from build123d import *

# Parameters (mm, degrees)
IZIM1_W                     = 500
IZIM1_H                     = 300
Y_KSEKLIK_EKSTR_ZYON1_DEPTH = 3


with BuildPart() as part:
    # Çizim1 → Yükseklik-Ekstrüzyon1 (new body)
    with BuildSketch(Plane.XY):
        with Locations((250, -150)):
            Rectangle(IZIM1_W, IZIM1_H)
        with BuildLine():
            Line((50, -40), (50, -120))
            ThreePointArc((50, -120), (45, -125), (40, -120))
            Line((40, -120), (40, -40))
            ThreePointArc((40, -40), (45, -35), (50, -40))
        make_face(mode=Mode.SUBTRACT)
        with BuildLine():
            Line((87.272727273, -40), (87.272727273, -120))
            ThreePointArc((87.272727273, -120), (82.272727273, -125), (77.272727273, -120))
            Line((77.272727273, -120), (77.272727273, -40))
            ThreePointArc((77.272727273, -40), (82.272727273, -35), (87.272727273, -40))
        make_face(mode=Mode.SUBTRACT)
        with BuildLine():
            Line((124.545454545, -40), (124.545454545, -120))
            ThreePointArc((124.545454545, -120), (119.545454545, -125), (114.545454545, -120))
            Line((114.545454545, -120), (114.545454545, -40))
            ThreePointArc((114.545454545, -40), (119.545454545, -35), (124.545454545, -40))
        make_face(mode=Mode.SUBTRACT)
        with BuildLine():
            Line((161.818181818, -40), (161.818181818, -120))
            ThreePointArc((161.818181818, -120), (156.818181818, -125), (151.818181818, -120))
            Line((151.818181818, -120), (151.818181818, -40))
            ThreePointArc((151.818181818, -40), (156.818181818, -35), (161.818181818, -40))
        make_face(mode=Mode.SUBTRACT)
        with BuildLine():
            Line((199.090909091, -40), (199.090909091, -120))
            ThreePointArc((199.090909091, -120), (194.090909091, -125), (189.090909091, -120))
            Line((189.090909091, -120), (189.090909091, -40))
            ThreePointArc((189.090909091, -40), (194.090909091, -35), (199.090909091, -40))
        make_face(mode=Mode.SUBTRACT)
        with BuildLine():
            Line((236.363636364, -40), (236.363636364, -120))
            ThreePointArc((236.363636364, -120), (231.363636364, -125), (226.363636364, -120))
            Line((226.363636364, -120), (226.363636364, -40))
            ThreePointArc((226.363636364, -40), (231.363636364, -35), (236.363636364, -40))
        make_face(mode=Mode.SUBTRACT)
        with BuildLine():
            Line((273.636363636, -40), (273.636363636, -120))
            ThreePointArc((273.636363636, -120), (268.636363636, -125), (263.636363636, -120))
            Line((263.636363636, -120), (263.636363636, -40))
            ThreePointArc((263.636363636, -40), (268.636363636, -35), (273.636363636, -40))
        make_face(mode=Mode.SUBTRACT)
        with BuildLine():
            Line((310.909090909, -40), (310.909090909, -120))
            ThreePointArc((310.909090909, -120), (305.909090909, -125), (300.909090909, -120))
            Line((300.909090909, -120), (300.909090909, -40))
            ThreePointArc((300.909090909, -40), (305.909090909, -35), (310.909090909, -40))
        make_face(mode=Mode.SUBTRACT)
        with BuildLine():
            Line((348.181818182, -40), (348.181818182, -120))
            ThreePointArc((348.181818182, -120), (343.181818182, -125), (338.181818182, -120))
            Line((338.181818182, -120), (338.181818182, -40))
            ThreePointArc((338.181818182, -40), (343.181818182, -35), (348.181818182, -40))
        make_face(mode=Mode.SUBTRACT)
        with BuildLine():
            Line((385.454545455, -40), (385.454545455, -120))
            ThreePointArc((385.454545455, -120), (380.454545455, -125), (375.454545455, -120))
            Line((375.454545455, -120), (375.454545455, -40))
            ThreePointArc((375.454545455, -40), (380.454545455, -35), (385.454545455, -40))
        make_face(mode=Mode.SUBTRACT)
        with BuildLine():
            Line((422.727272727, -40), (422.727272727, -120))
            ThreePointArc((422.727272727, -120), (417.727272727, -125), (412.727272727, -120))
            Line((412.727272727, -120), (412.727272727, -40))
            ThreePointArc((412.727272727, -40), (417.727272727, -35), (422.727272727, -40))
        make_face(mode=Mode.SUBTRACT)
        with BuildLine():
            Line((460, -40), (460, -120))
            ThreePointArc((460, -120), (455, -125), (450, -120))
            Line((450, -120), (450, -40))
            ThreePointArc((450, -40), (455, -35), (460, -40))
        make_face(mode=Mode.SUBTRACT)
        with BuildLine():
            Line((87.272727273, -180), (87.272727273, -260))
            ThreePointArc((87.272727273, -260), (82.272727273, -265), (77.272727273, -260))
            Line((77.272727273, -260), (77.272727273, -180))
            ThreePointArc((77.272727273, -180), (82.272727273, -175), (87.272727273, -180))
        make_face(mode=Mode.SUBTRACT)
        with BuildLine():
            Line((124.545454545, -180), (124.545454545, -260))
            ThreePointArc((124.545454545, -260), (119.545454545, -265), (114.545454545, -260))
            Line((114.545454545, -260), (114.545454545, -180))
            ThreePointArc((114.545454545, -180), (119.545454545, -175), (124.545454545, -180))
        make_face(mode=Mode.SUBTRACT)
        with BuildLine():
            Line((161.818181818, -180), (161.818181818, -260))
            ThreePointArc((161.818181818, -260), (156.818181818, -265), (151.818181818, -260))
            Line((151.818181818, -260), (151.818181818, -180))
            ThreePointArc((151.818181818, -180), (156.818181818, -175), (161.818181818, -180))
        make_face(mode=Mode.SUBTRACT)
        with BuildLine():
            Line((199.090909091, -180), (199.090909091, -260))
            ThreePointArc((199.090909091, -260), (194.090909091, -265), (189.090909091, -260))
            Line((189.090909091, -260), (189.090909091, -180))
            ThreePointArc((189.090909091, -180), (194.090909091, -175), (199.090909091, -180))
        make_face(mode=Mode.SUBTRACT)
        with BuildLine():
            Line((236.363636364, -180), (236.363636364, -260))
            ThreePointArc((236.363636364, -260), (231.363636364, -265), (226.363636364, -260))
            Line((226.363636364, -260), (226.363636364, -180))
            ThreePointArc((226.363636364, -180), (231.363636364, -175), (236.363636364, -180))
        make_face(mode=Mode.SUBTRACT)
        with BuildLine():
            Line((273.636363636, -180), (273.636363636, -260))
            ThreePointArc((273.636363636, -260), (268.636363636, -265), (263.636363636, -260))
            Line((263.636363636, -260), (263.636363636, -180))
            ThreePointArc((263.636363636, -180), (268.636363636, -175), (273.636363636, -180))
        make_face(mode=Mode.SUBTRACT)
        with BuildLine():
            Line((310.909090909, -180), (310.909090909, -260))
            ThreePointArc((310.909090909, -260), (305.909090909, -265), (300.909090909, -260))
            Line((300.909090909, -260), (300.909090909, -180))
            ThreePointArc((300.909090909, -180), (305.909090909, -175), (310.909090909, -180))
        make_face(mode=Mode.SUBTRACT)
        with BuildLine():
            Line((348.181818182, -180), (348.181818182, -260))
            ThreePointArc((348.181818182, -260), (343.181818182, -265), (338.181818182, -260))
            Line((338.181818182, -260), (338.181818182, -180))
            ThreePointArc((338.181818182, -180), (343.181818182, -175), (348.181818182, -180))
        make_face(mode=Mode.SUBTRACT)
        with BuildLine():
            Line((385.454545455, -180), (385.454545455, -260))
            ThreePointArc((385.454545455, -260), (380.454545455, -265), (375.454545455, -260))
            Line((375.454545455, -260), (375.454545455, -180))
            ThreePointArc((375.454545455, -180), (380.454545455, -175), (385.454545455, -180))
        make_face(mode=Mode.SUBTRACT)
        with BuildLine():
            Line((422.727272727, -180), (422.727272727, -260))
            ThreePointArc((422.727272727, -260), (417.727272727, -265), (412.727272727, -260))
            Line((412.727272727, -260), (412.727272727, -180))
            ThreePointArc((412.727272727, -180), (417.727272727, -175), (422.727272727, -180))
        make_face(mode=Mode.SUBTRACT)
        with BuildLine():
            Line((460, -180), (460, -260))
            ThreePointArc((460, -260), (455, -265), (450, -260))
            Line((450, -260), (450, -180))
            ThreePointArc((450, -180), (455, -175), (460, -180))
        make_face(mode=Mode.SUBTRACT)
        with BuildLine():
            Line((50, -180), (50, -260))
            ThreePointArc((50, -260), (45, -265), (40, -260))
            Line((40, -260), (40, -180))
            ThreePointArc((40, -180), (45, -175), (50, -180))
        make_face(mode=Mode.SUBTRACT)
    extrude(amount=Y_KSEKLIK_EKSTR_ZYON1_DEPTH)


solid = part.part
Can you work these out from the model? Positions are in its coordinate system, mm. Give positions to 0.01 mm unless a question says otherwise; leave off trailing zeros. Write each loop counter-clockwise with the first axis right and the second up, starting at its lowest first coordinate (ties: lowest second). Pieces come first, ordered by that corner, then holes. Notation, with made-up numbers: M 66.25,15 L 115.25,15 A27 ccw 115.25,43 Z; hole C -34,76.25 d8. An arc over 180 degrees is marked long. Answer in a Markdown table with one row per item. Add a question column.
Item 1: Please list where this line runs through material, in increasing order: L1, parallel to Y at x = 230.5, z = 1.4.
Item 2: Imagine slicing it at B-B, the plane y = -197.5. State how many separate pieces and enclosed holes the cut face has, plus the area to 3 significant figures.
Item 3: Imagine slicing it at A-A, the plane x = 455. Write out the boundary of the cut face in (y, z), plus the area to 3 significant figures.
Evaluation:
| question | item | result |
|---|---|---|
| 1 | L1 | y = -300 to -264.92, -175.08 to -124.92, -35.08 to 0 |
| 2 | separate pieces | 13 |
| 2 | enclosed holes | 0 |
| 2 | area | 1,140 mm² |
| 3 | outline | M -300,0 L -265,0 L -265,3 L -300,3 Z; M -175,0 L -125,0 L -125,3 L -175,3 Z; M -35,0 L 0,0 L 0,3 L -35,3 Z |
| 3 | area | 360 mm² |
